from build123d import *

# Parameters (mm, degrees)
BASPROSKE_W        = 62
BASPROSKE_H        = 28
TOOTHCUT_DEPTH     = 74.566296631
TEETHCUTS_COUNT    = 26
TEETHCUTS_ANGLE    = 346.153846154
BORSKE_R           = 0.4
BORE_DEPTH         = 62.0000508
CUT_EXTRUDE1_DEPTH = 74.51313205


with BuildPart() as part:
    # BasProSke → Base-Revolve (revolve)
    with BuildSketch(Plane(origin=(0, 0, 0), x_dir=(1, 0, 0), z_dir=(0, 1, 0)), mode=Mode.PRIVATE) as base_revolve_sk:
        with Locations((31, 14)):
            Rectangle(BASPROSKE_W, BASPROSKE_H)
    revolve(base_revolve_sk.sketch.rotate(Axis((-10, 0, 0), (1, 0, 0)), 180), axis=Axis((-10, 0, 0), (1, 0, 0)))

    # TooCutSke → ToothCut (cut, through all)
    with BuildSketch(Plane(origin=(0, 0, 0), x_dir=(0, 0, -1), z_dir=(1, 0, 0))):
        with BuildLine():
            ThreePointArc((0.939856059, 23.480197435), (0, 23.499), (-0.939856059, 23.480197435))
            ThreePointArc((-0.939856059, 23.480197435), (-1.620069556, 25.791248201), (-2.813767052, 27.883790276))
            ThreePointArc((-2.813767052, 27.883790276), (0, 28.0254), (2.813767052, 27.883790276))
            ThreePointArc((2.813767052, 27.883790276), (1.620069556, 25.791248201), (0.939856059, 23.480197435))
        make_face()
    toothcut = extrude(amount=TOOTHCUT_DEPTH, mode=Mode.SUBTRACT)

    # TeethCuts: ToothCut ×26 about axis
    teethcuts_axis = Axis((-10, 0, 0), (1, 0, 0))
    for i in range(1, TEETHCUTS_COUNT):
        add(toothcut.rotate(teethcuts_axis, i * TEETHCUTS_ANGLE / (TEETHCUTS_COUNT - 1)), mode=Mode.SUBTRACT)

    # BorSke → Bore (cut, symmetric)
    with BuildSketch(Plane(origin=(0, 0, 0), x_dir=(0, 0, -1), z_dir=(1, 0, 0))):
        with Locations(Location((0, 0, 0), (0, 0, 180))):
            Circle(BORSKE_R)
    extrude(amount=BORE_DEPTH, both=True, mode=Mode.SUBTRACT)

    # Sketch1 → Cut-Extrude1 (cut, through all)
    with BuildSketch(Plane(origin=(62, 0, 0), x_dir=(0, 0, -1), z_dir=(1, 0, 0))):
        with BuildLine():
            Line((-5, 19), (5, 19))
            Line((5, 19), (5, 15.324490204))
            ThreePointArc((5, 15.324490204), (0.82110488, -15.994457499), (-5, 15.061208451))
            Line((-5, 15.061208451), (-5, 19))
        make_face()
    extrude(amount=-CUT_EXTRUDE1_DEPTH, mode=Mode.SUBTRACT)


solid = part.part
Input: part model. Units: mm. Frame: model coordinates. A direction names the side the tool comes from. Round coordinates to 2 decimals unless told otherwise and drop trailing zeros. Write each loop counter-clockwise with the first axis right and the second up, starting at its lowest first coordinate (ties: lowest second). Pieces come first, ordered by that corner, then holes.
1) Reachability of faces 1 (the cylindrical face through (30.566, -4.693, 25.366)), 2 (the cylindrical face through (30.57, -10.67, -23.55)), 3 (the cylindrical face through (30.57, 7.63, -24.71)) from +Z, -Z, +X, -X, +Y, -Y: full face, straight path, thin tool, end or side. Return the list, or none.
2) Contact query for flat-ended pins moving along their axis: P1, Ø2, axis at x = 39, z = 16, coming from the +Y side; P2, Ø6, axis at x = 53.5, y = -12.5, coming from the +Z side; P3, Ø5, axis at x = 44.5, z = -1.5, coming from the -Y side; P4, Ø10, axis at x = 44, y = 8, coming from the -Z side. Output: stop coordinate, or through.
3) Draft query along Y for faces 4 (the cylindrical face through (30.57, 25.81, -1.63)), 5 (the cylindrical face through (30.57, 13.31, 22.1)), 6 (the cylindrical face through (30.566, -24.669, 7.757)). Return one class per face: pulls with the +Y half, pulls with the -Y half, needs draft (parallel to the pull), parting line crosses it, or undercut.
4) Ray query, L1, parallel to Y at x = 13, z = 0 (3 decimals); L2, parallel to Z at x = 25, y = 0; L3, parallel to Y at x = 56.5, z = 19. Return the intervals inside material, ascending.
5) Cut plane A-A (y = -11). Return the cut outline in (x, z).
Geometry says:
1. face 1: +Z, +X, -X
1. face 2: -Z, +X, -X
1. face 3: +X, -X
2. P1: stops at y = 23.37
2. P2: stops at z = 25.06
2. P3: stops at y = -27.86
2. P4: stops at z = -27.32
3. face 4: pulls with the +Y half
3. face 5: undercut
3. face 6: pulls with the -Y half
4. L1: y = -23.499 to -15.995, 19 to 23.499
4. L2: z = -28 to -16.4, 15.6 to 28
4. L3: y = -18.53 to -14.32, -13.83 to 13.83, 14.32 to 18.53
5. outline: (0, -23.88) - (62, -23.88) - (62, -12.02) - (0, -12.02) - close; (0, 11.22) - (62, 11.22) - (62, 23.88) - (0, 23.88) - close
